Geometry check sheet. Reference: the model listing, model coordinates, mm. A direction names the side the tool comes from. Round coordinates to 2 decimals unless told otherwise and drop trailing zeros. Order: outer loops, then holes, each group sorted by start corner. A loop starts at its lowest first (then second) coordinate and runs counter-clockwise, first axis right, second up.
(1) Sectioned sample at D-D (x = 4). Record the boundary of the cut face in (y, z).
(2) Sectioned sample at B-B (y = 3). Record the boundary of the cut face in (x, z).
(3) Sectioned sample at A-A (z = 16). Record the boundary of the cut face in (x, y).
(4) Set-up check for faces 1 (the face through (23, -39.573, 45)), 2 (the face through (-1, -7, 13)), 3 (the face through (-26, -39.573, 45)): record each of +Z, -Z, +X, -X, +Y, -Y from which the full face is reachable in a straight line by a thin tool's end or side.
(5) Go/stop test with flat-tipped pins: pin 1 (6 mm diameter, centred on x = 20.5, z = 40.5, fed in from -Y); pin 2 (1 mm diameter, centred on x = 5.5, z = 51.5, fed in from -Y); pin 3 (19 mm diameter, centred on x = 0, y = -14, fed in from +Z); pin 4 (20 mm diameter, centred on y = -7.57, z = 36, fed in from +X). Record where each tip stops, or that it passes through.
(6) Material ranges on line 1 along X through (y, z) = (-25.5, 45); line 2 along Y through (x, z) = (-23, 53); line 3 along X through (y, z) = (-42, 51.5), recorded low to high.
(7) Sectioned sample at C-C (z = 36). Record the boundary of the cut face in (x, y), plus the area to 3 significant figures.
(8) Release check for a two-part mould opening along Y. For faces 4 (the face through (-1, 11.32, 42)), 5 (the face through (-12.09, -54, 33)), 6 (the face through (-0.94, -65.94, 44.62)) record: +Y half, -Y half, draft (parallel to the pull), parting line (faces both ways), or undercut.
from build123d import *

# Parameters (mm, degrees)
F0_W      = 75.9807191789
F0_H      = 63.8928804547
F1_DEPTH  = 72
F2_T      = -13
F3_R      = 12.5
F4_DEPTH  = 100
F6_DEPTH  = 56
F8_DEPTH  = 52
F10_DEPTH = 25
F12_DEPTH = 25


with BuildPart() as f1:
    # F0 (on Top) → F1 (new body)
    with BuildSketch(Plane.XY):
        with Locations((-0.7195156068, -7.6268529519)):
            Rectangle(F0_W, F0_H)
    extrude(amount=F1_DEPTH)

    # F2
    f2_openings = [f1.faces().sort_by_distance(p)[0] for p in [
        (-0.719516, -7.626853, 72),
    ]]
    offset(amount=F2_T, openings=f2_openings)

    # F3 (on face) → F4 (cut)
    with BuildSketch(Plane.YZ.offset(37.2708439827)):
        with Locations((-7.5732931793, 36)):
            Circle(F3_R)
    extrude(amount=-F4_DEPTH, mode=Mode.SUBTRACT)

    # F5 (on face) → F6 (join)
    with BuildSketch(Plane.XZ.offset(39.5732931793)):
        Polygon((-38.7098751962, 0), (37.2708439827, 0), (37.2708439827, 18), (10.2804843932, 18), (-11.7195156068, 18), (-38.7098751962, 18), align=None)
    extrude(amount=F6_DEPTH)

    # F7 (on face) → F8 (join)
    with BuildSketch(Plane.XZ.offset(39.5732931793)):
        Polygon((-0.7098751962, 72), (-12.0902489871, 72), (-12.0902489871, 18), (9.9097510129, 18), (9.9097510129, 72), align=None)
    extrude(amount=F8_DEPTH)

    # F9 (on face) → F10 (cut)
    with BuildSketch(Plane.YZ.offset(9.9097510129)):
        Polygon((-91.5732931793, 72), (-91.5732931793, 18), (-39.5732931793, 72), align=None)
    extrude(amount=-F10_DEPTH, mode=Mode.SUBTRACT)

    # F11 (on face) → F12 (cut)
    with BuildSketch(Plane.XY.offset(18)):
        with BuildLine():
            ThreePointArc((37.2708439827, -57.5732931793), (-0.7195156068, -95.5636527687), (-38.7098751962, -57.5732931793))
            Line((-38.7098751962, -57.5732931793), (-38.7098751962, -95.5732931793))
            Line((-38.7098751962, -95.5732931793), (37.2708439827, -95.5732931793))
            Line((37.2708439827, -95.5732931793), (37.2708439827, -57.5732931793))
        make_face()
    extrude(amount=-F12_DEPTH, mode=Mode.SUBTRACT)


solid = f1.part
Answer below:
1. outline: (-95.27, 0) - (24.32, 0) - (24.32, 72) - (11.32, 72) - (11.32, 13) - (-26.57, 13) - (-26.57, 72) - (-39.57, 72) - (-91.57, 18) - (-95.27, 18) - close
2. outline: (-38.71, 0) - (37.27, 0) - (37.27, 29.33) - (24.27, 29.33) - (24.27, 13) - (-25.71, 13) - (-25.71, 29.33) - (-38.71, 29.33) - close; (-38.71, 42.67) - (-25.71, 42.67) - (-25.71, 72) - (-38.71, 72) - close; (24.27, 42.67) - (37.27, 42.67) - (37.27, 72) - (24.27, 72) - close
3. outline: (-38.71, -57.57) arc R37.99 ccw to (37.27, -57.57) - (37.27, 24.32) - (-38.71, 24.32) - close; hole (-25.71, -26.57) - (24.27, -26.57) - (24.27, 11.32) - (-25.71, 11.32) - close
4. face 1: +Z, +X, -Y
4. face 2: +Z
4. face 3: +Z, -X, -Y
5. pin 1: stops at y = -39.57
5. pin 2: stops at y = -59.8
5. pin 3: stops at z = 13
5. pin 4: passes through
6. line 1: x = -38.71 to -25.71, 24.27 to 37.27
6. line 2: y = -39.57 to -26.57, 11.32 to 24.32
6. line 3: x = -12.09 to 9.91
7. outline: (-38.71, -39.57) - (-12.09, -39.57) - (-12.09, -74.24) - (9.91, -74.24) - (9.91, -39.57) - (37.27, -39.57) - (37.27, -20.07) - (24.27, -20.07) - (24.27, -26.57) - (-25.71, -26.57) - (-25.71, -20.07) - (-38.71, -20.07) - close; (-38.71, 4.93) - (-25.71, 4.93) - (-25.71, 11.32) - (24.27, 11.32) - (24.27, 4.93) - (37.27, 4.93) - (37.27, 24.32) - (-38.71, 24.32) - close
7. area: 3,070 mm2
8. face 4: undercut
8. face 5: draft
8. face 6: -Y half
